Part model, mm, in its own coordinate system. A direction names the side the tool comes from. Coordinates: 2 decimals unless noted, no trailing zeros. Write each loop counter-clockwise with the first axis right and the second up, starting at its lowest first coordinate (ties: lowest second). Pieces come first, ordered by that corner, then holes. Notation, with made-up numbers: M 43.25,88 L 87.25,88 A26 cw 87.25,126 Z; hole C 88.25,1.5 d6. An arc over 180 degrees is marked long. Use a Markdown table: item, result. Add a question column.
Q1. Pin check, flat tips, straight feed: pin 1 Ø2.5 at (x, z) = (23.5, 2.5) entering from +Y; pin 2 Ø6 at (y, z) = (21, 4) entering from +X; pin 3 Ø0.5 at (x, y) = (3, 25.5) entering from -Z. Stop position of each tip, or through.
Q2. Slice it at A-A on x = 15. Write the cut outline in (y, z), then the cut area to 3 significant figures.
Q3. Slice it at B-B on z = 1.75. Write the cut outline in (x, y), then the cut area to 3 significant figures.
Q4. Tool access for faces 5 (the cylindrical face through (5.43, 25.75, 4.55)), 6 (the flat face through (20, 17, 5)), 7 (the flat face through (4.2, 25.5, 7)), 8 (the flat face through (3, 23, 3)), 9 (the flat face through (-2, 13, 5)): list every direction of +Z, -Z, +X, -X, +Y, -Y with a clear straight run to the whole face (end or side of a thin tool).
Q5. Mould opens along X. For faces 1 (the flat face through (3.8, 26, 3.2)), 2 (the flat face through (-5, 14, 5)), 3 (the cylindrical face through (23.21, 14.01, 4.66)), 4 (the flat face through (4, 25.5, 5)) say: released by +X, released by -X, zero draft, split by the parting line, or undercut.
Q6. Wall check: L1, parallel to X at y = 14.05, z = 5; L2, parallel to Z at x = 4, y = 25.7; L3, parallel to X at y = 25.7, z = 5. Give the ranges that are in metal, low to high. Write a range as from..to.
Q7. Slice it at D-D on z = 5. Count the separate pieces of the cut face and the enclosed holes in it, then the cut area to 3 significant figures.
Q8. Slice it at C-C on x = 20.5. Write the cut outline in (y, z).
Autodesk Inventor part; units mm, degrees
ref_plane "YZ Plane" through (0, 0, 0) normal (1, 0, 0) x (0, 1, 0)
ref_plane "XZ Plane" through (0, 0, 0) normal (0, 1, 0) x (-1, 0, 0)
ref_plane "XY Plane" through (0, 0, 0) normal (0, 0, 1) x (1, 0, 0)
sketch "Sketch1" plane through (0, 0, 0) normal (0, 0, 1) x (1, 0, 0)
  line L0 (0, 0) -> (20, 0)
  line L1 (20, 0) -> (20, 20)
  line L2 (20, 20) -> (0, 20)
  line L3 (0, 20) -> (0, 0)
  dimension "d0" = 20
  dimension "d1" = 20
extrude "Extrusion1" add sketch "Sketch1" along normal blind 10
sketch "Sketch2" plane through (20, 0, 0) normal (1, 0, 0) x (0, 0, -1)
  line L0 (0, 0) -> (0, 20)
  line L1 (0, 15) -> (-10, 15)
  line L2 (-10, 15) -> (-10, 13)
  line L3 (-10, 13) -> (0, 13)
  line L4 (0, 13) -> (0, 15)
  dimension "d4" = 10
  dimension "d5" = 2
extrude "Extrusion2" add sketch "Sketch2" along normal blind 5
sketch "Sketch3" plane through (0, 0, 0) normal (-1, 0, 0) x (0, 0, 1)
  line L0 (10, 15) -> (10, 13)
  line L1 (0, 15) -> (10, 15)
  line L2 (10, 15) -> (10, 13)
  line L3 (10, 13) -> (0, 13)
  line L4 (0, 13) -> (0, 15)
  point P0 (0, 0)
  dimension "d8" = 2
extrude "Extrusion3" add sketch "Sketch3" along normal blind 5
sketch "Sketch4" plane through (20, 15, 10) normal (0, 1, 0) x (1, 0, 0)
  circle A0 centre (-23.5755, 5) radius 0.5
  line L0 (0, 10) -> (-20, 10)
  line L1 (-10, 10) -> (-10, 0.1248)
  line L2 (-10, 0.1248) -> (-10, 10)
  circle A1 centre (3.5755, 5) radius 0.5
  dimension "d11" = 1
extrude "Extrusion4" cut sketch "Sketch4" against normal through all
sketch "Sketch5" plane through (0, 20, 0) normal (0, 1, 0) x (1, 0, 0)
  circle A0 centre (4, -5) radius 3.9548
  point P0 (0, 0)
extrude "Extrusion5" add sketch "Sketch5" along normal blind 3
sketch "Sketch6" plane through (4, 23, 5) normal (0, 1, 0) x (1, 0, 0)
  circle A0 centre (0, 0) radius 2
  point P0 (-4, 5)
  dimension "d16" = 4
extrude "Extrusion6" add sketch "Sketch6" along normal blind 2
sketch "Sketch7" plane through (4, 25, 5) normal (0, 1, 0) x (1, 0, 0)
  circle A0 centre (0, 0) radius 2
  line L0 (0, 2) -> (13, 2)
  line L1 (15, 0) -> (15, 0)
  line L2 (13, -2) -> (0, -2)
  line L3 (0, -2) -> (0, 2)
  line L4 (0, 2) -> (-13, 2)
  line L5 (-15, 0) -> (-15, 0)
  line L6 (-13, -2) -> (0, -2)
  line L7 (0, -2) -> (0, 2)
  arc A1 (-13, 2) -> (-15, 0) centre (-13, 0) ccw
  arc A2 (-15, 0) -> (-13, -2) centre (-13, 0) ccw
  arc A3 (13, -2) -> (15, 0) centre (13, 0) ccw
  arc A4 (15, 0) -> (13, 2) centre (13, 0) ccw
  point P0 (-4, 5)
  point P1 (15, -2)
  point P2 (-15, -2)
  point P3 (0, -2)
  point P4 (15, 0)
  dimension "d19" = 15
  dimension "d20" = 15
  dimension "d21" = 2
extrude "Extrusion7" add sketch "Sketch7" along normal blind 1
sketch "Sketch8" plane through (4, 26, 5) normal (0, 1, 0) x (1, 0, 0)
  circle A0 centre (0, 0) radius 1.5
  point P0 (-4, 5)
  dimension "d24" = 3
extrude "Extrusion8" cut sketch "Sketch8" against normal blind 0.5
properties part number "servo"
Recorded:
| question | item | result |
|---|---|---|
| 1 | pin 1 | y = 15 |
| 1 | pin 2 | x = 20 |
| 1 | pin 3 | z = 3 |
| 2 | outline | M 0,0 L 20,0 L 20,10 L 0,10 Z; M 25,3 L 26,3 L 26,7 L 25,7 Z |
| 2 | area | 204 mm² |
| 3 | outline | M -5,13 L 0,13 L 0,0 L 20,0 L 20,13 L 25,13 L 25,15 L 20,15 L 20,20 L 6.25,20 L 6.25,23 L 1.75,23 L 1.75,20 L 0,20 L 0,15 L -5,15 Z |
| 3 | area | 434 mm² |
| 4 | face 5 | +Y |
| 4 | face 6 | +Z, -Z, +X, +Y |
| 4 | face 7 | +Z, +X, -X, +Y |
| 4 | face 8 | none |
| 4 | face 9 | +Z, -Z, -X, -Y |
| 5 | face 1 | zero draft |
| 5 | face 2 | released by -X |
| 5 | face 3 | undercut |
| 5 | face 4 | undercut |
| 6 | L1 | -5..-4.08, -3.08..23.08, 24.08..25 |
| 6 | L2 | 3..3.5, 6.5..7 |
| 6 | L3 | -11..2.5, 5.5..19 |
| 7 | separate pieces | 3 |
| 7 | enclosed holes | 0 |
| 7 | area | 476 mm² |
| 8 | outline | M 13,0 L 15,0 L 15,10 L 13,10 Z |
